Read the model definition and answer for the solid it produces. Units are mm, in the model's axes. A direction names the side the tool comes from. Coordinates: 2 decimals unless noted, no trailing zeros. Order: outer loops, then holes, each group sorted by start corner. A loop starts at its lowest first (then second) coordinate and runs counter-clockwise, first axis right, second up.
```python
from build123d import *

# Parameters (mm, degrees)
BOSS_EXTRUDE1_DEPTH = 3.13
BOSS_EXTRUDE2_DEPTH = 2.71
BOSS_EXTRUDE3_DEPTH = 2.28
SKETCH6_W           = 7.320164266
SKETCH6_H           = 2.185


with BuildPart() as part:
    # Sketch1 → Boss-Extrude1 (new body)
    with BuildSketch(Plane.XY):
        with BuildLine():
            Line((-7.335, 0), (-7.335, -9.395))
            Line((-7.335, -9.395), (7.335, -9.395))
            Line((7.335, -9.395), (7.335, 0))
            ThreePointArc((7.335, 0), (0, 7.335), (-7.335, 0))
        make_face()
    extrude(amount=BOSS_EXTRUDE1_DEPTH)

    # Sketch2 → Boss-Extrude2 (add)
    with BuildSketch(Plane(origin=(0, 0, 0), x_dir=(-1, 0, 0), z_dir=(0, 0, -1))):
        with BuildLine():
            Line((-4.435, -0.4), (-4.435, -6.755))
            Line((-4.435, -6.755), (4.435, -6.755))
            Line((4.435, -6.755), (4.435, -0.4))
            ThreePointArc((4.435, -0.4), (0, 4.035), (-4.435, -0.4))
        make_face()
    extrude(amount=BOSS_EXTRUDE2_DEPTH)

    # Sketch3 → Boss-Extrude3 (add)
    with BuildSketch(Plane(origin=(0, 0, -2.71), x_dir=(-1, 0, 0), z_dir=(0, 0, -1))):
        with BuildLine():
            Line((-7.235, -13.005), (7.235, -13.005))
            Line((7.235, -13.005), (7.235, -1.32))
            ThreePointArc((7.235, -1.32), (0, 5.915), (-7.235, -1.32))
            Line((-7.235, -1.32), (-7.235, -13.005))
        make_face()
    extrude(amount=BOSS_EXTRUDE3_DEPTH)

    # Sketch5 → Revolve1 (revolve)
    with BuildSketch(Plane(origin=(0, 0, 0), x_dir=(0, 0, -1), z_dir=(1, 0, 0)), mode=Mode.PRIVATE) as revolve1_sk:
        Polygon((4.99, 3.57), (9.99, 3.57), (9.99, 2.815), (24.99, 2.28), (24.99, -1.32), (4.99, -1.32), align=None)
    revolve(revolve1_sk.sketch.rotate(Axis((0, -1.32, -24.99), (0, 0, -1)), 180), axis=Axis((0, -1.32, -24.99), (0, 0, -1)))

    # Sketch6 → Revolve2 (revolve)
    with BuildSketch(Plane(origin=(0, 0, 0), x_dir=(0, 0, -1), z_dir=(1, 0, 0))):
        with Locations((-6.790082133, -0.2275)):
            Rectangle(SKETCH6_W, SKETCH6_H)
    revolve(axis=Axis((0, -1.32, 10.450164266), (0, 0, 1)))


solid = part.part
```
1) A cutting plane is placed at B-B, the plane x = 0. Determine the outline of the cut face in (y, z) (3 decimals).
A:
outline: (-13.005, -4.99) - (-6.21, -4.99) - (-6.21, -9.99) - (-5.455, -9.99) - (-4.92, -24.99) - (2.28, -24.99) - (2.815, -9.99) - (3.57, -9.99) - (3.57, -4.99) - (5.915, -4.99) - (5.915, -2.71) - (4.035, -2.71) - (4.035, 0) - (7.335, 0) - (7.335, 3.13) - (0.865, 3.13) - (0.865, 10.45) - (-3.505, 10.45) - (-3.505, 3.13) - (-9.395, 3.13) - (-9.395, 0) - (-6.755, 0) - (-6.755, -2.71) - (-13.005, -2.71) - close
2) Straight lines are drawn through the part: line 1 (Z direction, x = -5.5, y = -3); line 2 (Z direction, x = 5.5, y = -11.75); line 3 (Z direction, x = 2.75, y = -2.5). For each, find the intervals that lie inside material, in ascending order.
A:
line 1: z = -4.99 to -2.71, 0 to 3.13
line 2: z = -4.99 to -2.71
line 3: z = -24.99 to 3.13
3) Determine the mould class of faces 6 (the flat face through (-2, -3, 3.13)), 7 (the cylindrical face through (0.161, 7.333, 1.543)), 8 (the flat face through (0, -8, -2.71)) for opening direction Z: pulls with the +Z half, pulls with the -Z half, needs draft (parallel to the pull), parting line crosses it, or undercut.
A:
face 6: pulls with the +Z half
face 7: needs draft
face 8: undercut
4) A cutting plane is placed at C-C, the plane z = 6.5. Determine the outline of the cut face in (x, y) (3 decimals), and give its area (3 significant figures).
A:
outline: circle Ø4.37 at (0, -1.32)
area: 15.0 mm2
5) A cutting plane is placed at D-D, the plane z = -6.5. Determine the outline of the cut face in (x, y).
A:
outline: circle Ø9.78 at (0, -1.32)
6) Flat-ended cylindrical pins translate along their axes: pin 1 Ø0.7 at (y, z) = (-7.5, -4) entering from -X (3 decimals); pin 2 Ø2 at (y, z) = (-3, -1.5) entering from -X (3 decimals); pin 3 Ø1.6 at (x, z) = (-3, 1) entering from -Y (3 decimals); pin 4 Ø5 at (x, z) = (-0.5, 4) entering from +Y (3 decimals). Find the tip coordinate at first contact, or state that the pin passes through.
A:
pin 1: stops at x = -7.235
pin 2: stops at x = -4.435
pin 3: stops at y = -9.395
pin 4: stops at y = 7.335
7) A cutting plane is placed at A-A, the plane y = 5. Determine the outline of the cut face in (x, z), and give its area (3 significant figures).
A:
outline: (-5.37, 0) - (5.37, 0) - (5.37, 3.13) - (-5.37, 3.13) - close; (-3.52, -4.99) - (3.52, -4.99) - (3.52, -2.71) - (-3.52, -2.71) - close
area: 49.7 mm2
8) Which of the six approach directions +Z, -Z, +X, -X, +Y, -Y give full straight-line access (tool end or side, diameter ignored) to faces 1 (the cylindrical face through (-0.159, 5.913, -3.834)), 2 (the flat face through (-1, 3, -9.99)), 3 (the flat face through (0, -9.395, 2)), 4 (the flat face through (4.435, -4, -1)), 5 (the cylindrical face through (2.133, -1.794, 6.739))?
A:
face 1: -Z, +Y
face 2: -Z
face 3: +Z, +X, -X, -Y
face 4: +X, +Y, -Y
face 5: +Z
